The figure shows three views and two pictorial views of one solid part (mm, origin at its lowest corner). Answer the questions. A direction names the side the tool comes from. Coordinates: 2 decimals unless noted, no trailing zeros. Loops run counter-clockwise (first coordinate to the right, second up) from the corner with the lowest first, then second, coordinate; pieces in that order, holes last.
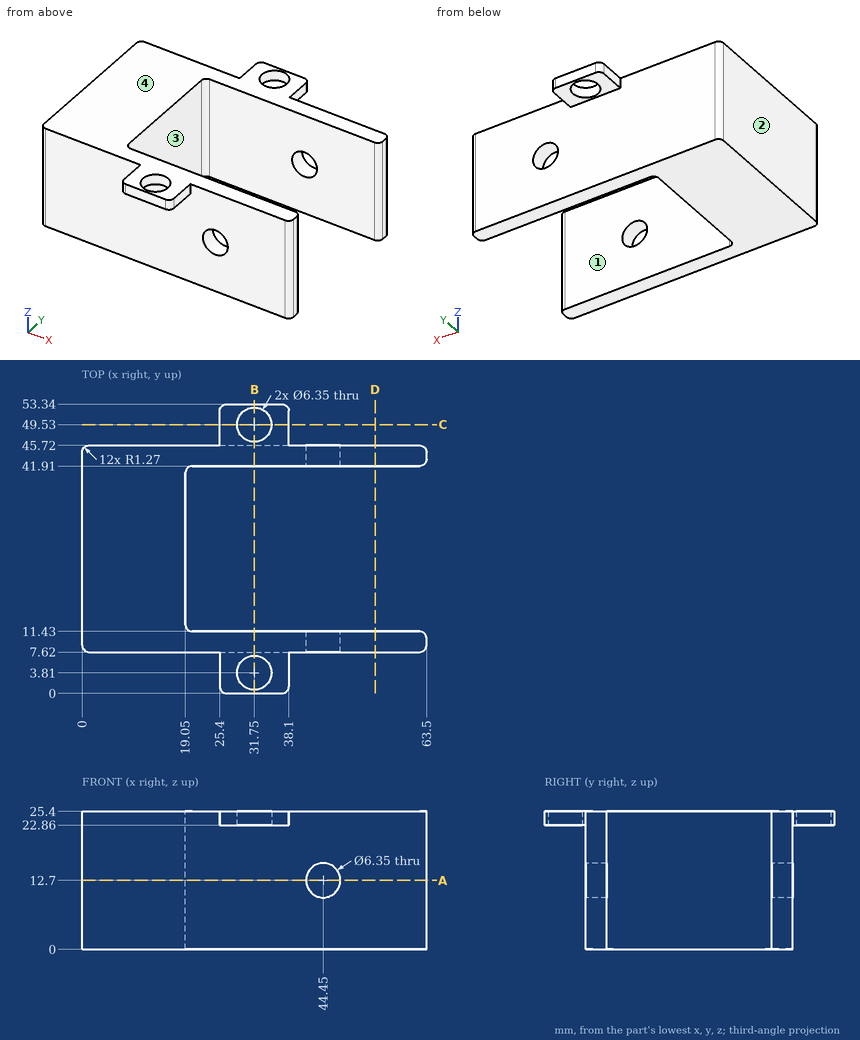
Q1. Straight lines are drawn through the part: probe 1 along Y at (x, z) = (31.75, 24.05) (3 decimals); probe 2 along Z at (x, y) = (44.45, 44.45) (3 decimals); probe 3 along Y at (x, z) = (53.5, 19.75). For each, find the intervals that lie inside material, in ascending order.
Findings below:
probe 1: y = 0 to 0.635, 6.985 to 11.43, 41.91 to 46.355, 52.705 to 53.34
probe 2: z = 0 to 9.525, 15.875 to 25.4
probe 3: y = 7.62 to 11.43, 41.91 to 45.72
Q2. Flat-ended cylindrical pins translate along their axes: pin 1 Ø6 at (x, z) = (9, 10.5) entering from -Y; pin 2 Ø1.3 at (y, z) = (49, 24) entering from -X; pin 3 Ø8 at (x, z) = (50, 7) entering from +Y; pin 4 Ø8.5 at (x, y) = (31.75, 49.53) entering from +Z. Find the tip coordinate at first contact, or state that the pin passes through.
Findings below:
pin 1: stops at y = 7.62
pin 2: stops at x = 25.4
pin 3: stops at y = 45.72
pin 4: stops at z = 25.4
Q3. A cutting plane is placed at A-A (z = 12.7). Give the vertices of the cut face in (x, y) (3 decimals).
Findings below:
outline: (0, 8.89) arc R1.27 ccw to (1.27, 7.62) - (41.275, 7.62) - (41.275, 11.43) - (20.32, 11.43) arc R1.27 cw to (19.05, 12.7) - (19.05, 40.64) arc R1.27 cw to (20.32, 41.91) - (41.275, 41.91) - (41.275, 45.72) - (1.27, 45.72) arc R1.27 ccw to (0, 44.45) - close; (47.625, 7.62) - (62.23, 7.62) arc R1.27 ccw to (63.5, 8.89) - (63.5, 10.16) arc R1.27 ccw to (62.23, 11.43) - (47.625, 11.43) - close; (47.625, 41.91) - (62.23, 41.91) arc R1.27 ccw to (63.5, 43.18) - (63.5, 44.45) arc R1.27 ccw to (62.23, 45.72) - (47.625, 45.72) - close
Q4. A cutting plane is placed at D-D (x = 54). Give the vertices of the cut face in (y, z), then the cut area to 3 significant figures.
Findings below:
outline: (7.62, 0) - (11.43, 0) - (11.43, 25.4) - (7.62, 25.4) - close; (41.91, 0) - (45.72, 0) - (45.72, 25.4) - (41.91, 25.4) - close
area: 194 mm2
Q5. A cutting plane is placed at C-C (y = 49.53). Give the vertices of the cut face in (x, z) (3 decimals).
Findings below:
outline: (25.4, 22.86) - (28.575, 22.86) - (28.575, 25.4) - (25.4, 25.4) - close; (34.925, 22.86) - (38.1, 22.86) - (38.1, 25.4) - (34.925, 25.4) - close
Q6. A cutting plane is placed at B-B (x = 31.75). Give the vertices of the cut face in (y, z) (3 decimals).
Findings below:
outline: (0, 22.86) - (0.635, 22.86) - (0.635, 25.4) - (0, 25.4) - close; (6.985, 22.86) - (7.62, 22.86) - (7.62, 0) - (11.43, 0) - (11.43, 25.4) - (6.985, 25.4) - close; (41.91, 0) - (45.72, 0) - (45.72, 22.86) - (46.355, 22.86) - (46.355, 25.4) - (41.91, 25.4) - close; (52.705, 22.86) - (53.34, 22.86) - (53.34, 25.4) - (52.705, 25.4) - close
Q7. Which of the six approach directions +Z, -Z, +X, -X, +Y, -Y give full straight-line access (tool end or side, diameter ignored) to the marked faces 1 and 2?
Findings below:
face 1: +Z, -Z, +X
face 2: +Z, -Z, -X, +Y, -Y
Q8. Determine the mould class of the marked faces 3 and 4 for opening direction Y: +Y half, -Y half, draft (parallel to the pull), parting line (faces both ways), or undercut.
Findings below:
face 3: undercut
face 4: draft
